CAD build for the part. Positions are in the model's coordinates, mm. Coordinates: 2 decimals unless noted, no trailing zeros. Write each loop counter-clockwise with the first axis right and the second up, starting at its lowest first coordinate (ties: lowest second). Pieces come first, ordered by that corner, then holes. Notation, with made-up numbers: (-17, 17.25) - (6, 17.25) arc R17 cw to (6, 44.25) - close; hole circle Ø5 at (-28, 26.5). An arc over 180 degrees is marked (long way). Answer in a Markdown table with one row per item. Add a question column.
Q1. Band-saw the part on B-B (x = -118). List the corners of the cut face in (y, z).
Q2. Band-saw the part on A-A (y = -444.5). List the corners of the cut face in (x, z), and give its area (3 significant figures).
Q3. Two-plate mould, pull along X, no slides. Class faces 1 (the cylindrical face through (-101.95, -406.724, 6.439)), 2 (the flat face through (-2, 7, 0)): +X half, -X half, draft (parallel to the pull), parting line (faces both ways), or undercut.
Q4. Drill centre lines: line 1 along Y through (x, z) = (-146.05, 3.5); line 2 along Y through (x, z) = (0, 4); line 3 along Y through (x, z) = (-101.5, 9). Where is each one in solid material? Low to high. Write a range as from..to.
Q5. Pin check, flat tips, straight feed: pin 1 (3 mm diameter, centred on x = 0, y = -527.05, fed in from +Z); pin 2 (4 mm diameter, centred on y = -57.5, z = 6, fed in from +X). Stop position of each tip, or through.
Q6. Band-saw the part on D-D (y = -185). List the corners of the cut face in (x, z), and give its area (3 significant figures).
Q7. Band-saw the part on C-C (z = 6.5). State how many separate pieces and enclosed holes the cut face has, and give its area (3 significant figures).
```python
from build123d import *

# Parameters (mm, degrees)
F1_DEPTH = 12.7
F2_R     = 1.7272
F2_R_2   = 38.1
F3_DEPTH = 12.7
F4_R     = 1.7272
F5_DEPTH = 12.7


with BuildPart() as f1:
    # F0 (on Top) → F1 (new body)
    with BuildSketch(Plane.XY):
        Polygon((-152.4, 355.6), (-152.4, -355.6), (-177.8, -355.6), (-177.8, -533.4), (177.8, -533.4), (177.8, -355.6), (152.4, -355.6), (152.4, 355.6), (177.8, 355.6), (177.8, 533.4), (-177.8, 533.4), (-177.8, 355.6), align=None)
    extrude(amount=F1_DEPTH)

    # F2 (on face) → F3 (cut, through all)
    with BuildSketch(Plane.XY.offset(12.7)):
        with Locations((-145.37171, 492.881133)):
            Circle(F2_R)
        with Locations((-48.609445, 492.881133)):
            Circle(F2_R)
        with Locations((-145.37171, 396.118867)):
            Circle(F2_R)
        with Locations((-48.609445, 396.118867)):
            Circle(F2_R)
        with Locations((-145.37171, -492.881133)):
            Circle(F2_R)
        with Locations((-145.37171, -396.118867)):
            Circle(F2_R)
        with Locations((-48.609445, -492.881133)):
            Circle(F2_R)
        with Locations((-48.609445, -396.118867)):
            Circle(F2_R)
        with Locations((-96.990578, -444.5)):
            Circle(F2_R_2)
        with Locations((96.990578, -444.5)):
            Circle(F2_R_2)
        with Locations((-96.990578, 444.5)):
            Circle(F2_R_2)
        with Locations((96.990578, 444.5)):
            Circle(F2_R_2)
        with Locations((-10.31875, 366.786655)):
            Circle(F2_R)
        with Locations((10.31875, 398.536655)):
            Circle(F2_R)
        with Locations((10.31875, 366.786655)):
            Circle(F2_R)
        with Locations((-10.31875, 398.536655)):
            Circle(F2_R)
    extrude(amount=-F3_DEPTH, mode=Mode.SUBTRACT)

    # F4 (on face) → F5 (cut, through all)
    with BuildSketch(Plane.XY.offset(12.7)):
        with Locations((0, 263.525)):
            Circle(F4_R)
        with Locations((-146.05, 0)):
            Circle(F4_R)
        with Locations((146.05, 0)):
            Circle(F4_R)
        with Locations((0, 527.05)):
            Circle(F4_R)
        with Locations((0, -263.525)):
            Circle(F4_R)
        with Locations((0, -527.05)):
            Circle(F4_R)
    extrude(amount=-F5_DEPTH, mode=Mode.SUBTRACT)


solid = f1.part
```
Checked values:
| question | item | result |
|---|---|---|
| 1 | outline | (-533.4, 0) - (-476.28, 0) - (-476.28, 12.7) - (-533.4, 12.7) - close; (-412.72, 0) - (412.72, 0) - (412.72, 12.7) - (-412.72, 12.7) - close; (476.28, 0) - (533.4, 0) - (533.4, 12.7) - (476.28, 12.7) - close |
| 2 | outline | (-177.8, 0) - (-135.09, 0) - (-135.09, 12.7) - (-177.8, 12.7) - close; (-58.89, 0) - (58.89, 0) - (58.89, 12.7) - (-58.89, 12.7) - close; (135.09, 0) - (177.8, 0) - (177.8, 12.7) - (135.09, 12.7) - close |
| 2 | area | 2,580 mm² |
| 3 | face 1 | undercut |
| 3 | face 2 | draft |
| 4 | line 1 | y = -533.4..-494.47, -491.29..-397.71, -394.53..-1.73, 1.73..394.53, 397.71..491.29, 494.47..533.4 |
| 4 | line 2 | y = -533.4..-528.78, -525.32..-265.25, -261.8..261.8, 265.25..525.32, 528.78..533.4 |
| 4 | line 3 | y = -533.4..-482.33, -406.67..406.67, 482.33..533.4 |
| 5 | pin 1 | passes through |
| 5 | pin 2 | stops at x = 152.4 |
| 6 | outline | (-152.4, 0) - (152.4, 0) - (152.4, 12.7) - (-152.4, 12.7) - close |
| 6 | area | 3,870 mm² |
| 7 | separate pieces | 1 |
| 7 | enclosed holes | 22 |
| 7 | area | 325,000 mm² |
